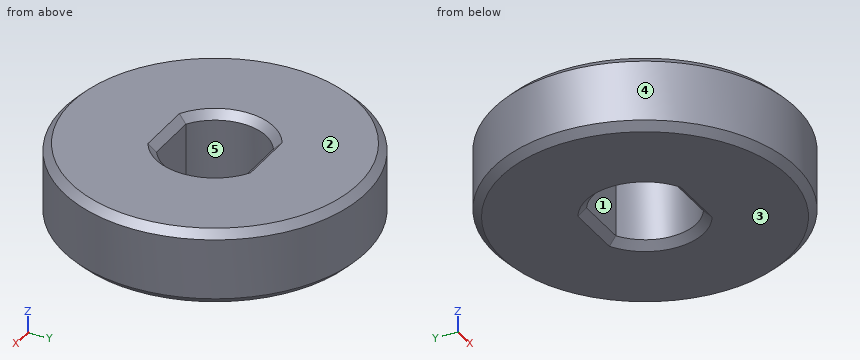
from build123d import *

# Parameters (mm, degrees)
SKETCH1_R           = 10
BOSS_EXTRUDE1_DEPTH = 5
CHAMFER1_SIZE       = 0.5


with BuildPart() as part:
    # Sketch1 → Boss-Extrude1 (new body)
    with BuildSketch(Plane.XY):
        Circle(SKETCH1_R)
        with BuildLine():
            Line((-1.774823935, 2.9), (1.774823935, 2.9))
            ThreePointArc((1.774823935, 2.9), (3.4, 0), (1.774823935, -2.9))
            Line((1.774823935, -2.9), (-1.774823935, -2.9))
            ThreePointArc((-1.774823935, -2.9), (-3.4, 0), (-1.774823935, 2.9))
        make_face(mode=Mode.SUBTRACT)
    extrude(amount=BOSS_EXTRUDE1_DEPTH)

    # Chamfer1
    chamfer1_edges = [part.edges().sort_by_distance(p)[0] for p in [
        (3.4, 0, 5),
        (0, 2.9, 5),
        (-10, 0, 0),
        (-10, 0, 5),
        (-3.4, 0, 0),
        (0, -2.9, 0),
        (3.4, 0, 0),
        (0, 2.9, 0),
        (-3.4, 0, 5),
        (0, -2.9, 5),
    ]]
    chamfer(chamfer1_edges, length=CHAMFER1_SIZE)


solid = part.part
Check sheet for the modelled part. Datum: model origin and axes. Units: mm. Face numbers are marked on the shaded views. A direction names the side the tool comes from. Give positions to 0.01 mm unless a question says otherwise; leave off trailing zeros. Loops run counter-clockwise (first coordinate to the right, second up) from the corner with the lowest first, then second, coordinate; pieces in that order, holes last. Notation, with made-up numbers: M -18,-22.75 L 20,-22.75 A9 ccw 20,-14.75 Z; hole C 17.25,74.25 d9. An arc over 180 degrees is marked long. Use a Markdown table: item, result. Add a question column.
Q1. Sectioned sample at A-A, the plane x = 0. Record the cut outline in (y, z).
Q2. Tool access check on the marked faces 1 and 2. Record the directions out of +Z, -Z, +X, -X, +Y, -Y that give a thin tool (end or side, any length) a straight path to the whole face; none if there is none.
Q3. Sectioned sample at C-C, the plane z = 1.7. Record the cut outline in (x, y), then the cut area to 3 significant figures.
Q4. Go/stop test with flat-tipped pins: pin 1 (3 mm diameter, centred on x = 6, z = 1, fed in from -Y); pin 2 (2 mm diameter, centred on x = -3.5, z = 4.5, fed in from +Y); pin 3 (1 mm diameter, centred on y = -4.5, z = 2, fed in from -X). Record where each tip stops, or that it passes through.
Q5. Sectioned sample at B-B, the plane y = 0. Record the cut outline in (x, z).
Q6. Scan lines: line 1 along X through (y, z) = (-1, 4.25); line 2 along X through (y, z) = (2.5, 3.9); line 3 along Y through (x, z) = (6.25, 2.6). Record each from-to range of solid material in increasing order. Write a range as [from, to].
Q7. Mould release check, pull along X, two halves, no side actions. Record for the marked faces 3, 4 and 5: pulls with the +X half, pulls with the -X half, needs draft (parallel to the pull), parting line crosses it, or undercut.
Verdict:
| question | item | result |
|---|---|---|
| 1 | outline | M -10,0.5 L -9.5,0 L -3.4,0 L -2.9,0.5 L -2.9,4.5 L -3.4,5 L -9.5,5 L -10,4.5 Z; M 2.9,0.5 L 3.4,0 L 9.5,0 L 10,0.5 L 10,4.5 L 9.5,5 L 3.4,5 L 2.9,4.5 Z |
| 2 | face 1 | +Z, -Z |
| 2 | face 2 | +Z, +X, -X, +Y, -Y |
| 3 | outline | C 0,0 d20; hole M -1.77,-2.9 L 1.77,-2.9 A3.4 ccw 1.77,2.9 L -1.77,2.9 A3.4 ccw Z |
| 3 | area | 280 mm^2 |
| 4 | pin 1 | y = -8.93 |
| 4 | pin 2 | y = 9.68 |
| 4 | pin 3 | x = -9.17 |
| 5 | outline | M -10,0.5 L -9.5,0 L -3.9,0 L -3.4,0.5 L -3.4,4.5 L -3.9,5 L -9.5,5 L -10,4.5 Z; M 3.4,0.5 L 3.9,0 L 9.5,0 L 10,0.5 L 10,4.5 L 9.5,5 L 3.9,5 L 3.4,4.5 Z |
| 6 | line 1 | [-9.95, -3.25], [3.25, 9.95] |
| 6 | line 2 | [-9.68, -2.3], [2.3, 9.68] |
| 6 | line 3 | [-7.81, 7.81] |
| 7 | face 3 | needs draft |
| 7 | face 4 | parting line crosses it |
| 7 | face 5 | undercut |
